The model under review builds one solid part; all positions refer to its coordinate system, in mm. A direction names the side the tool comes from. Coordinates: 2 decimals unless noted, no trailing zeros. Write each loop counter-clockwise with the first axis right and the second up, starting at its lowest first coordinate (ties: lowest second). Pieces come first, ordered by that corner, then holes. Notation, with made-up numbers: (43.5, 24.5) - (76.5, 24.5) arc R36 ccw to (76.5, 58.5) - close; hole circle Ø10 at (57, 22). An arc over 180 degrees is marked (long way). Use one line per item in the form item = value. Start each with the question number.
Autodesk Inventor part; units mm, degrees
ref_plane "YZ Plane" through (0, 0, 0) normal (1, 0, 0) x (0, 1, 0)
ref_plane "XZ Plane" through (0, 0, 0) normal (0, 1, 0) x (-1, 0, 0)
ref_plane "XY Plane" through (0, 0, 0) normal (0, 0, 1) x (1, 0, 0)
sketch "Sketch1" plane through (0, 0, 0) normal (0, 0, 1) x (1, 0, 0)
  line L0 (-16, 12.5) -> (-13, 12.5)
  line L1 (-13, 12.5) -> (-13, -9.5)
  line L2 (-13, -9.5) -> (13, -9.5)
  line L3 (13, -9.5) -> (13, 12.5)
  line L4 (13, 12.5) -> (16, 12.5)
  line L5 (16, 12.5) -> (16, -12.5)
  line L6 (16, -12.5) -> (-16, -12.5)
  line L7 (-16, -12.5) -> (-16, 12.5)
  point P0 (0, 0)
  dimension "d0" = 3
  dimension "d2" = 3
  dimension "d3" = 25
  dimension "d4" = 32
  dimension "d5" = 16
  dimension "d7" = 12.5
  dimension "d8" = 3
  dimension "d95" = 25
extrude "Extrusion1" add sketch "Sketch1" against normal blind 660.4
sketch "Sketch5" plane through (16, -12.5, 0) normal (1, 0, 0) x (0, 0, -1)
  circle A0 centre (16, 15.5) radius 3.175
  circle A1 centre (120.7333, 15.5) radius 3.175
  circle A2 centre (225.4667, 15.5) radius 3.175
  circle A3 centre (330.2, 15.5) radius 3.175
  circle A4 centre (434.9333, 15.5) radius 3.175
  circle A5 centre (539.6667, 15.5) radius 3.175
  circle A6 centre (644.4, 15.5) radius 3.175
  line L0 (0, 25) -> (0, 0)
  line L1 (660.4, 25) -> (660.4, 0)
  line L2 (0, 3) -> (660.4, 3)
  point P0 (0, 12.5)
  dimension "d56" = 6.35
  dimension "d58" = 6.35
  dimension "d59" = 6.35
  dimension "d61" = 6.35
  dimension "d63" = 6.35
  dimension "d64" = 6.35
  dimension "d65" = 6.35
  dimension "d68" = 16
  dimension "d78" = 660.4
  dimension "d79" = 16
  dimension "d80" = 628.4
  dimension "d81" = 104.7333
  dimension "d82" = 104.7333
  dimension "d83" = 104.7333
  dimension "d84" = 104.7333
  dimension "d85" = 104.7333
  dimension "d86" = 104.7333
  dimension "d94" = 12.5
hole "Hole1" at (16, 3, -644.4) at (16, 3, -539.6667) at (16, 3, -434.9333) at (16, 3, -330.2) at (16, 3, -225.4667) at (16, 3, -120.7333) at (16, 3, -16) direction (-1, 0, 0) diameter 6.35 depth 3 tip angle 118
sketch "Sketch6" plane through (-16, -12.5, 0) normal (-1, 0, 0) x (0, 0, 1)
  circle A0 centre (-16, 15.5) radius 3.175
  circle A1 centre (-644.4, 15.5) radius 3.175
  circle A2 centre (-644.4, 15.5) radius 3.175
  circle A3 centre (-16, 15.5) radius 3.175
  point P0 (0, 12.5)
hole "Hole2" at (-16, 3, -644.4) at (-16, 3, -16) direction (1, 0, 0) diameter 6.35 depth 3 tip angle 118
equation "\"d2\" = d0"
equation "\"d8\" = d0"
equation "\"d95\" = d3"
equation "\"d58\" = d56"
equation "\"d59\" = d58"
equation "\"d61\" = d60"
equation "\"d63\" = d62"
equation "\"d64\" = d63"
equation "\"d65\" = d64"
equation "\"d81\" = 0.166667 * d80"
equation "\"d82\" = d81"
equation "\"d83\" = d82"
equation "\"d84\" = d83"
equation "\"d85\" = d84"
equation "\"d60\" = d59"
equation "\"d62\" = d61"
properties part number "26in C-Channel Left" material "Aluminum 6061"
1. For faces 4 (the flat face through (-1, -10, 0)), 5 (the flat face through (-13, 2, -326)), list the 3-axis set-ups (+Z, -Z, +X, -X, +Y, -Y) from which the entire face can be reached by the end or side of a thin tool; tool diameter is ignored.
2. For P1, Ø8, axis at x = 4, z = -167, coming from the +Y side; P2, Ø5.5, axis at y = 3, z = -539.67, coming from the +X side; P3, Ø5, axis at y = 3, z = -644.4, coming from the +X side, all flat-tipped, find the tip position at first contact; note any pin that passes through.
3. Take a section at B-B (x = -1.5). State the section outline as (y, z) points, plus the area to 3 significant figures.
4. Take a section at A-A (z = -401.5). State the section outline as (x, y) points, plus the area to 3 significant figures.
5. For L1, parallel to Z at x = -14.9, y = 3 (3 decimals); L2, parallel to X at y = -6.5, z = -526.5; L3, parallel to Y at x = 14.6, z = -16 (3 decimals), list the stretches that pass through material, from the lowest coordinate up.
6. The part is to be moulded in two halves that separate along X. For faces 1 (the flat face through (-1, -10, -660.4)), 2 (the flat face through (-16, 0, -326)), 3 (the flat face through (13, 1, -326)), say which applies: released by +X, released by -X, zero draft, split by the parting line, or undercut.
Returned:
q1.face_4 = +Z, +X, -X, +Y, -Y
q1.face_5 = +Z, -Z, +Y
q2.P1 = -9.5
q2.P2 = -13
q2.P3 = through
q3.outline = (-12.5, -660.4) - (-9.5, -660.4) - (-9.5, 0) - (-12.5, 0) - close
q3.area = 1,980 mm²
q4.outline = (-16, -12.5) - (16, -12.5) - (16, 12.5) - (13, 12.5) - (13, -9.5) - (-13, -9.5) - (-13, 12.5) - (-16, 12.5) - close
q4.area = 228 mm²
q5.L1 = -660.4 to -647.575, -641.225 to -19.175, -12.825 to 0
q5.L2 = -16 to -13, 13 to 16
q5.L3 = -12.5 to -0.175, 6.175 to 12.5
q6.face_1 = zero draft
q6.face_2 = released by -X
q6.face_3 = undercut
